Build history of the part. All positions in model axes, mm. Coordinates: 2 decimals unless noted, no trailing zeros.
Item 1: Flat gauge pins, fed straight in: pin 1 (3 mm diameter, centred on y = -17, z = 17.5, fed in from +X); pin 2 (5 mm diameter, centred on y = -7, z = 23.5, fed in from +X); pin 3 (3 mm diameter, centred on x = -17, z = 22, fed in from -Y). Where does each tip first touch, or does it go through?
Item 2: Cut at A-A (z = 39.5). Count the separate pieces of the cut face and the enclosed holes in it, and give its area (3 significant figures).
Item 3: Mould opens along Y. For faces 1 (the face through (10.8, -20.76, 37.57)), 2 (the face through (-5.506, -24.796, 37.567)), 3 (the face through (0, 0, 76.2)) say: released by +Y, released by -Y, zero draft, split by the parting line, or undercut.
Item 4: Drill centre lines: line 1 along X through (y, z) = (-9, 63); line 2 along X through (y, z) = (7.5, 63); line 3 along Y through (x, z) = (4.5, 53.5). Where is each one in solid material? Low to high.
from build123d import *

# Parameters (mm, degrees)
F0_R     = 25.4
F0_R_2   = 23.4
F1_DEPTH = 76.2
F2_W     = 1
F2_H     = 24.8149117469
F2_W_2   = 24.8222645992
F2_H_2   = 1


with BuildPart() as f1:
    # F0 (on Top) → F1 (new body)
    with BuildSketch(Plane.XY):
        Circle(F0_R)
        Circle(F0_R_2, mode=Mode.SUBTRACT)
    extrude(amount=F1_DEPTH)

    # F2 (on Top) → F5 section 0
    with BuildSketch(Plane.XY):
        with Locations((0, -12.9074558734)):
            Rectangle(F2_W, F2_H)
    # F4 (on offset) → F5 section 1
    with BuildSketch(Plane.XY.offset(76.2)):
        Polygon((0, -0.7071067812), (-0.7071067812, 0), (-18.1997778835, -17.4926711023), (-17.4926711023, -18.1997778835), align=None)
    loft()

    # F2 (on Top) → F6 section 0
    with BuildSketch(Plane.XY):
        with Locations((-12.9111322996, 0)):
            Rectangle(F2_W_2, F2_H_2)
    # F4 (on offset) → F6 section 1
    with BuildSketch(Plane.XY.offset(76.2)):
        Polygon((-17.4616031125, 18.1687098937), (-18.1687098937, 17.4616031125), (-0.7071067812, 0), (0, 0.7071067812), align=None)
    loft()

    # F2 (on Top) → F7 section 0
    with BuildSketch(Plane.XY):
        with Locations((0, 12.9074558734)):
            Rectangle(F2_W, F2_H)
    # F4 (on offset) → F7 section 1
    with BuildSketch(Plane.XY.offset(76.2)):
        Polygon((17.4926711023, 18.1997778835), (0, 0.7071067812), (0.7071067812, 0), (18.1997778835, 17.4926711023), align=None)
    loft()

    # F2 (on Top) → F8 section 0
    with BuildSketch(Plane.XY):
        with Locations((12.9111322996, 0)):
            Rectangle(F2_W_2, F2_H_2)
    # F4 (on offset) → F8 section 1
    with BuildSketch(Plane.XY.offset(76.2)):
        Polygon((0.7071067812, 0), (0, -0.7071067812), (17.4616031125, -18.1687098937), (18.1687098937, -17.4616031125), align=None)
    loft()

    # F4 (on offset) → F9 section 0
    with BuildSketch(Plane.XY.offset(76.2)):
        Polygon((0, 0.7071067812), (-0.7071067812, 0), (0, -0.7071067812), (0.7071067812, 0), align=None)
    # F2 (on Top) → F9 section 1
    with BuildSketch(Plane.XY):
        Rectangle(F2_W, F2_H_2)
    loft()


solid = f1.part
Filled sheet:
1. pin 1: stops at x = 20.12
1. pin 2: stops at x = 25
1. pin 3: stops at y = -20.12
2. separate pieces: 2
2. enclosed holes: 1
2. area: 392 mm2
3. face 1: undercut
3. face 2: split by the parting line
3. face 3: zero draft
4. line 1: x = -23.75 to -21.6, -7.54 to -6.33, 10.9 to 12.46, 21.6 to 23.75
4. line 2: x = -24.27 to -22.17, -10.52 to -8.95, 5.18 to 6.39, 22.17 to 24.27
4. line 3: y = -25 to -22.96, -3.36 to -2.26, 6.32 to 8.09, 22.96 to 25
